Part model, mm, in its own coordinate system. A direction names the side the tool comes from. Coordinates: 2 decimals unless noted, no trailing zeros. Loops run counter-clockwise (first coordinate to the right, second up) from the corner with the lowest first, then second, coordinate; pieces in that order, holes last.
Autodesk Inventor part; units mm, degrees
ref_plane "Work Plane1" through (29, 0, 0) normal (0, -1, 0) x (1, 0, 0)
ref_plane "YZ Plane" through (0, 0, 0) normal (1, 0, 0) x (0, 1, 0)
ref_plane "XZ Plane" through (0, 0, 0) normal (0, 1, 0) x (-1, 0, 0)
sketch "Sketch1" plane through (0, 0, 0) normal (0, 0, 1) x (1, 0, 0)
  line L0 (-0.6667, 0) -> (35, 0)
  line L1 (35, 0) -> (35, 1.5)
  line L2 (35, 1.5) -> (17, 1.5)
  line L3 (17, 1.5) -> (16.6932, 1.5)
  line L4 (16.6932, 1.5) -> (0, 1.5)
  line L5 (0, 1.5) -> (0, 2.75)
  line L6 (0, 2.75) -> (-3, 2.75)
  line L7 (-3, 2.75) -> (-3, 1.4434)
  line L8 (-3, 1.4434) -> (-1.5, 1.4434)
  line L9 (-1.5, 1.4434) -> (-0.6667, 0)
  line L10 (-9.6, 0) -> (36.6, 0)
  line L11 (0, -0.55) -> (0, 3.3)
  line L12 (17, 1.5) -> (0, 1.5) construction
  dimension "d1" = 18
  dimension "d2" = 0.3068
  dimension "d3" = 3
  dimension "d4" = 1.5
  dimension "d5" = 60
  dimension "d6" = 3
  dimension "d7" = 3
  dimension "d8" = 2.8868
  dimension "d9" = 5.5
  dimension "d26" = 35
revolve "Body" add sketch "Sketch1" angle 360 about axis through (-0.6667, 0, 0) along (1, 0, 0)
sketch "Sketch2" plane through (-3, 0, 0) normal (-1, 0, 0) x (0, 0, 1)
  circle A0 centre (0, 0) radius 1.4434
  line L0 (0, -3.85) -> (0, 3.85)
  line L1 (-3.85, 0) -> (3.85, 0)
  line L2 (1.4434, 0) -> (0.7217, -1.25)
  line L3 (0.7217, -1.25) -> (-0.7217, -1.25)
  line L4 (-0.7217, -1.25) -> (-1.4434, 0)
  line L5 (-1.4434, 0) -> (-0.7217, 1.25)
  line L6 (-0.7217, 1.25) -> (0.7217, 1.25)
  line L7 (0.7217, 1.25) -> (1.4434, 0)
extrude "Slot" add sketch "Sketch2" against normal up to next contours L7 A0 | A0 L2 | L6 L0 A0 | A0 L0 L3 | L0 L6 A0 | A0 L3 L0 | L4 A0 | A0 L5
fillet "Fillet1" radius 0.3 1 edges at (-3, -2.75, 0)
thread "Thread"
chamfer "Chamfer1" distance 0.3067 distance2 0.3067 1 edges at (35, -1.5, 0) measured on face at (35, -0.8773, -0.3972)
ref_plane "Work Plane1" through (29, 0, 0) normal (0, -1, 0) x (1, 0, 0)
fillet "Fillet2" radius 0.1 1 edges at (0, -1.5, 0)
equation "\"d1\" = GEL"
equation "\"d3\" = KOH"
equation "\"d4\" = INTI"
equation "\"d6\" = GD"
equation "\"d7\" = BDM"
equation "\"d8\" = 1.1547 * SW"
equation "\"d9\" = KOD"
equation "\"d26\" = NLG"
equation "\"d30\" = R"
equation "\"d17\" = RR"
equation "\"d13\" = GEL"
equation "\"d15\" = -0.5 * SPD + 0.5 * GD"
equation "\"d16\" = GUL"
equation "\"GD\" = NND"
equation "\"NLG\" = 35"
equation "\"GEL\" = 18"
equation "\"KOD\" = 5.5"
equation "\"KOH\" = 3"
equation "\"INTI\" = 1.5"
equation "\"GAL\" = 0.61345 * PTC"
equation "\"GUL\" = 0.61345 * PTC"
equation "\"BDM\" = NND"
equation "\"SW\" = 2.5"
equation "\"RR\" = 0.3"
equation "\"SPD\" = 2.38655"
equation "\"R\" = 0.1"
equation "\"TOA\" = 30deg"
equation "\"THREADDIA\" = 3"
equation "\"PTC\" = 0.5"
equation "\"NND\" = 3"
equation "\"E0\" = 1.155 * SW"
equation "\"GD1\" = THREADDIA - 1.2269 * PTC"
properties material "Steel, Mild"
Q1. Saw through at A-A (x = 22). List the corners of the cut face in (y, z).
Q2. Tool access for faces 1 (the flat face through (-2, -1.25, 0)), 2 (the cylindrical face through (17.15, -1.5, -0.07)), 3 (the flat face through (-3, -1.1, 1.1)): list every direction of +Z, -Z, +X, -X, +Y, -Y with a clear straight run to the whole face (end or side of a thin tool).
Q3. Mould opens along Z. For faces 4 (the cylindrical face through (-1.369, -0.596, 2.685)), 5 (the flat face through (35, 0, 0)), 6 (the flat face through (-2.21, -0.63, -1.08)) say: released by +Z, released by -Z, zero draft, split by the parting line, or undercut.
Q4. Drop flat-ended pins along their axis: P1, Ø0.7, axis at x = -2, z = -0.5, coming from the -Y side; P2, Ø1, axis at x = 25, z = 1, coming from the -Y side; P3, Ø3, axis at x = 9.5, y = 0.5, coming from the +Z side. Give the stop position or say it passes through.
Q5. Probe line 1 (X direction, y = 1.9, z = 0.45); line 2 (Y direction, x = 29, z = -0.4); line 3 (Z direction, x = 3, y = -0.2). List the from-to ranges inside material, lowest first.
Checked values:
1. outline: circle Ø3 at (0, 0)
2. face 1: -X
2. face 2: +X
2. face 3: +Z, -Z, -X, +Y, -Y
3. face 4: split by the parting line
3. face 5: zero draft
3. face 6: undercut
4. P1: stops at y = -2.75
4. P2: stops at y = -1.41
4. P3: stops at z = 1.5
5. line 1: x = -3 to 0
5. line 2: y = -1.45 to 1.45
5. line 3: z = -1.49 to 1.49
